Work out the finished part from the listing and answer in its coordinate system (mm). Round coordinates to 2 decimals unless told otherwise and drop trailing zeros. Loops run counter-clockwise (first coordinate to the right, second up) from the corner with the lowest first, then second, coordinate; pieces in that order, holes last.
from build123d import *

# Parameters (mm, degrees)
SKETCH_1_W = 0.061
SKETCH_1_H = 9
SKETCH_4_W = 6
SKETCH_4_H = 3.7


with BuildPart() as part:
    # 草图1 → 旋转2 (revolve)
    with BuildSketch(Plane.XY, mode=Mode.PRIVATE) as revolve_2_sk:
        with Locations((0, 4.5)):
            Rectangle(SKETCH_1_W, SKETCH_1_H)
    revolve(revolve_2_sk.sketch.rotate(Axis((-0.0305, 0, 0), (1, 0, 0)), 90), axis=Axis((-0.0305, 0, 0), (1, 0, 0)))  # turned: the seam where the file's is

    # 草图4 → 旋转3 (revolve)
    with BuildSketch(Plane.XY, mode=Mode.PRIVATE) as revolve_3_sk:
        with Locations((0, 10.85)):
            Rectangle(SKETCH_4_W, SKETCH_4_H)
    revolve(revolve_3_sk.sketch.rotate(Axis((-1.614212419, 0, 0), (1, 0, 0)), 90), axis=Axis((-1.614212419, 0, 0), (1, 0, 0)))  # turned: the seam where the file's is


solid = part.part
Item 1: Section D-D, the plane y = 10.75 is taken. Give the vertices of the cut face in (x, z), plus the area to 3 significant figures.
Item 2: Determine the mould class of faces 1 (the face through (-1.494, -6.083, -6.633)), 2 (the face through (1.536, -6.083, -6.633)), 3 (the face through (3, 3, 9)), 4 (the face through (0, 7.7, -10.1)) for opening direction Z: pulls with the +Z half, pulls with the -Z half, needs draft (parallel to the pull), parting line crosses it, or undercut.
Item 3: Section A-A, the plane z = 0 is taken. Give the vertices of the cut face in (x, y), plus the area to 3 significant figures.
Item 4: Section C-C, the plane x = 1.3 is taken. Give the vertices of the cut face in (y, z).
Item 5: Each of these flat-tipped pins is pushed along its axis until it touches: P1, Ø14.5, axis at y = 0, z = 0, coming from the +X side; P2, Ø12, axis at y = 1.5, z = -2, coming from the -X side; P3, Ø1.5, axis at x = -2, z = 5.5, coming from the +Y side. Where does it stop, or does it pass through?
Item 6: Straight lines are drawn through the part: line 1 (Y direction, x = 2.35, z = 0); line 2 (Y direction, x = 2.25, z = 6.25); line 3 (Z direction, x = 2.3, y = 8). For each, find the intervals that lie inside material, in ascending order.
Answer below:
1. outline: (-3, -6.76) - (3, -6.76) - (3, 6.76) - (-3, 6.76) - close
1. area: 81.1 mm2
2. face 1: undercut
2. face 2: undercut
2. face 3: needs draft
2. face 4: parting line crosses it
3. outline: (-3, -12.7) - (3, -12.7) - (3, -9) - (0.03, -9) - (0.03, 9) - (3, 9) - (3, 12.7) - (-3, 12.7) - (-3, 9) - (-0.03, 9) - (-0.03, -9) - (-3, -9) - close
3. area: 45.5 mm2
4. outline: circle Ø25.4 at (0, 0); hole circle Ø18 at (0, 0)
5. P1: stops at x = 0.03
5. P2: stops at x = -0.03
5. P3: stops at y = 11.78
6. line 1: y = -12.7 to -9, 9 to 12.7
6. line 2: y = -11.06 to -6.48, 6.48 to 11.06
6. line 3: z = -9.86 to -4.12, 4.12 to 9.86
